Check sheet for the modelled part. Datum: model origin and axes. Units: mm. A direction names the side the tool comes from. Give positions to 0.01 mm unless a question says otherwise; leave off trailing zeros. Loops run counter-clockwise (first coordinate to the right, second up) from the corner with the lowest first, then second, coordinate; pieces in that order, holes last.
Autodesk Inventor part; units mm, degrees
ref_plane "YZ Plane" through (0, 0, 0) normal (1, 0, 0) x (0, 1, 0)
ref_plane "XZ Plane" through (0, 0, 0) normal (0, 1, 0) x (-1, 0, 0)
ref_plane "XY Plane" through (0, 0, 0) normal (0, 0, 1) x (1, 0, 0)
sketch "Sketch1" plane through (0, 0, 0) normal (0, 1, 0) x (-1, 0, 0)
  circle A0 centre (0, 0) radius 19.05
  circle A1 centre (0, 0) radius 12.7
  circle A2 centre (0, 0) radius 4
  line L0 (12.7, 0) -> (11.2, 0)
  circle A3 centre (11.2, 0) radius 1.5
  line L1 (11.2, 1.5) -> (2.3814, 3.2139)
  line L2 (11.2, -1.5) -> (2.3814, -3.2139)
  circle A4 centre (0, 11.2) radius 1.5
  line L3 (-1.5, 11.2) -> (-3.2139, 2.3814)
  line L4 (1.5, 11.2) -> (3.2139, 2.3814)
  circle A5 centre (-11.2, 0) radius 1.5
  line L5 (-11.2, -1.5) -> (-2.3814, -3.2139)
  line L6 (-11.2, 1.5) -> (-2.3814, 3.2139)
  circle A6 centre (0, -11.2) radius 1.5
  line L7 (1.5, -11.2) -> (3.2139, -2.3814)
  line L8 (-1.5, -11.2) -> (-3.2139, -2.3814)
  line L9 (0, -19.05) -> (29.9563, -19.05)
  line L10 (29.9563, -19.05) -> (29.9563, 19.05)
  line L11 (29.9563, 19.05) -> (0, 19.05)
  line L12 (0, 19.05) -> (0, -19.05)
  point P0 (0, 12.7)
  point P1 (-12.7, 0)
  point P2 (0, -12.7)
  point P3 (-3.0784, -3.0784)
  point P4 (-3.0784, 3.0784)
  point P5 (3.0784, 3.0784)
  point P6 (3.0784, -3.0784)
  point P7 (0, 19.05)
  dimension "d2" = 38.1
  dimension "d3" = 25.4
  dimension "d4" = 8
  dimension "d5" = 1.5
  dimension "d6" = 360
extrude "Extrusion1" add sketch "Sketch1" along normal blind 2 contours A0 L12 A1 | A0 L11 L10 L9 | L12 A1 A0 | A4 L3 L6 A5 A1 | A1 A3 L1 L4 A4 | A6 L7 L2 A3 A1 | A1 A5 L5 L8 A6
sketch "Sketch2" plane through (0, 2, 0) normal (0, 1, 0) x (1, 0, 0)
  line L0 (0, 19.05) -> (-29.9563, 19.05)
  line L1 (-29.9563, -19.05) -> (0, -19.05)
  line L2 (0, -19.05) -> (0, 19.05)
  line L3 (0, 19.05) -> (-29.9563, 19.05)
  line L4 (-29.9563, 19.05) -> (-29.9563, -19.05)
  circle A0 centre (0, 0) radius 19.05
  point P0 (0, -19.05)
extrude "Extrusion2" add sketch "Sketch2" along normal blind 3
sketch "Sketch3" plane through (0, 0, 0) normal (0, -1, 0) x (1, 0, 0)
  point P0 (0, 0)
sketch "Sketch4" plane through (0, 5, 0) normal (0, 1, 0) x (1, 0, 0)
  line L0 (-29.9563, -19.05) -> (-24.9563, -19.05)
  line L1 (-24.9563, -19.05) -> (-24.9563, 18.9252)
  line L2 (-24.9563, 18.9252) -> (-29.9563, 18.9252)
  line L3 (-29.9563, 18.9252) -> (-29.9563, -19.05)
  point P0 (0, 0)
  dimension "d11" = 5
extrude "Extrusion3" add sketch "Sketch4" against normal blind 40.64
properties part number "turret y top"
(1) Section check D-D on z = -5.5. Record the boundary of the cut face in (x, y).
(2) Gauge pin test, flat ends, axial feed: pin 1 Ø1 at (y, z) = (-20, 3.5) entering from +X; pin 2 Ø5.5 at (x, y) = (-27.5, -13) entering from -Z; pin 3 Ø2 at (x, z) = (-16, -3) entering from -Y. Record the tip position at first contact, or that the pin passes through.
(3) Material ranges on line 1 (X direction, y = -22, z = -12.5); line 2 (Y direction, x = -11.5, z = -9.5); line 3 (Z direction, x = -25, y = -15), recorded low to high.
(4) Access from +Z, -Z, +X, -X, +Y, -Y to the whole of each face (thin tool, end or side, straight path). Record for faces 1 (the face through (-24.956, -18, 0)), 2 (the face through (-27, -18, -18.925)), 3 (the face through (-7.196, 0.986, 2.278)).
(5) Release check for a two-part mould opening along X. For faces 4 (the face through (-29.956, -16, 0)), 5 (the face through (-2.278, 0.986, -7.196)), 6 (the face through (-27, -35.64, 0)) record: pulls with the +X half, pulls with the -X half, needs draft (parallel to the pull), parting line crosses it, or undercut.
(6) Section check B-B on y = -32. Record the boundary of the cut face in (x, z), plus the area to 3 significant figures.
(7) Section check C-C on x = -23. Record the boundary of the cut face in (y, z), plus the area to 4 significant figures.
(8) Section check A-A on z = 0. Record the boundary of the cut face in (x, y).
Computed values:
1. outline: (-29.96, -35.64) - (-24.96, -35.64) - (-24.96, 0) - (-2.61, 0) - (-2.61, 2) - (2.61, 2) - (2.61, 0) - (18.24, 0) - (18.24, 5) - (-29.96, 5) - close
2. pin 1: stops at x = -24.96
2. pin 2: stops at z = -18.93
2. pin 3: stops at y = 0
3. line 1: x = -29.96 to -24.96
3. line 2: y = 0 to 5
3. line 3: z = -18.93 to 19.05
4. face 1: +Z, -Z, +X, -Y
4. face 2: -Z, +X, -X, -Y
4. face 3: -Y
5. face 4: pulls with the -X half
5. face 5: undercut
5. face 6: needs draft
6. outline: (-29.96, -18.93) - (-24.96, -18.93) - (-24.96, 19.05) - (-29.96, 19.05) - close
6. area: 190 mm2
7. outline: (0, -19.05) - (5, -19.05) - (5, 19.05) - (0, 19.05) - close
7. area: 190.5 mm2
8. outline: (-29.96, -35.64) - (-24.96, -35.64) - (-24.96, 0) - (-12.7, 0) - (-12.7, 2) - (12.7, 2) - (12.7, 0) - (19.05, 0) - (19.05, 5) - (-29.96, 5) - close
